from build123d import *

# Parameters (mm, degrees)
F0_R     = 12.7
F1_DEPTH = 241.3
F2_R     = 2.5527
F3_DEPTH = 15.24
F4_R     = 2.5527
F5_DEPTH = 15.24


with BuildPart() as f1:
    # F0 (on Right) → F1 (new body)
    with BuildSketch(Plane.YZ):
        Circle(F0_R)
    extrude(amount=F1_DEPTH)

    # F2 (on face) + F0 (on Right) → F3 (cut)
    with BuildSketch(Plane(origin=(0, 0, 0), x_dir=(0, -1, 0), z_dir=(-1, 0, 0))):
        Circle(F2_R)
    with BuildSketch(Plane.YZ):
        Circle(F0_R)
    extrude(amount=-F3_DEPTH, mode=Mode.SUBTRACT)

    # F4 (on face) → F5 (cut)
    with BuildSketch(Plane.YZ.offset(241.3)):
        Circle(F4_R)
    extrude(amount=-F5_DEPTH, mode=Mode.SUBTRACT)


solid = f1.part
Verification items for the finished model (mm, model axes). A direction names the side the tool comes from. Round coordinates to 2 decimals unless told otherwise and drop trailing zeros. Write each loop counter-clockwise with the first axis right and the second up, starting at its lowest first coordinate (ties: lowest second). Pieces come first, ordered by that corner, then holes.
(1) Section check D-D (y = 10.5). Enter the section's corners in (x, z), plus the area to 3 significant figures.
Returned:
outline: (0, -7.14) - (241.3, -7.14) - (241.3, 7.14) - (0, 7.14) - close
area: 3,450 mm2
(2) Material ranges on line 1 (Z direction, x = 6.25, y = 0); line 2 (Y direction, x = 45, z = -0.75); line 3 (X direction, y = 2, z = -0.5), recorded low to high.
Returned:
line 1: z = -12.7 to -2.55, 2.55 to 12.7
line 2: y = -12.68 to 12.68
line 3: x = 15.24 to 226.06
(3) Section check A-A (z = 0). Enter the section's corners in (x, y), plus the area to 3 significant figures.
Returned:
outline: (0, -12.7) - (241.3, -12.7) - (241.3, -2.55) - (226.06, -2.55) - (226.06, 2.55) - (241.3, 2.55) - (241.3, 12.7) - (0, 12.7) - (0, 2.55) - (15.24, 2.55) - (15.24, -2.55) - (0, -2.55) - close
area: 5,970 mm2
(4) Access from +Z, -Z, +X, -X, +Y, -Y to the whole of each face (thin tool, end or side, straight path). Record for faces 4 (the flat face through (0, 3, 0)), 5 (the cylindrical face through (7.513, -2.435, 0.767)), 6 (the flat face through (226.06, 0, 0)).
Returned:
face 4: +Z, -Z, -X, +Y, -Y
face 5: -X
face 6: +X
(5) Section check C-C (x = 87.5). Enter the section's corners in (y, z), plus the area to 3 significant figures.
Returned:
outline: circle Ø25.4 at (0, 0)
area: 507 mm2
(6) Depth check by flat-ended pin: pin 1 Ø5 at (x, z) = (51, 7.5) entering from +Y; pin 2 Ø4.5 at (y, z) = (0, 0) entering from -X; pin 3 Ø1.5 at (y, z) = (0.5, 0.5) entering from +X. Enter the tip coordinate at first touch or a pass-through.
Returned:
pin 1: stops at y = 11.67
pin 2: stops at x = 15.24
pin 3: stops at x = 226.06
(7) Mould release check, pull along Y, two halves, no side actions. Record for faces 1 (the cylindrical face through (233.787, 2.435, 0.767)), 2 (the flat face through (241.3, 3, 0)), 3 (the cylindrical face through (118.96, -2.75, -12.4)): pulls with the +Y half, pulls with the -Y half, needs draft (parallel to the pull), parting line crosses it, or undercut.
Returned:
face 1: undercut
face 2: needs draft
face 3: parting line crosses it
